Source: three-view drawing plus pictorial views. Frame: mm from the lowest corner of the part. A direction names the side the tool comes from. Give positions to 0.01 mm unless a question says otherwise; leave off trailing zeros. Loops run counter-clockwise (first coordinate to the right, second up) from the corner with the lowest first, then second, coordinate; pieces in that order, holes last.
1. First-contact query: P1, Ø6, axis at x = 48.5, y = 18, coming from the +Z side; P2, Ø1.5, axis at x = 25, y = 12.5, coming from the +Z side; P3, Ø2, axis at x = 42, z = 2, coming from the -Y side; P4, Ø2, axis at x = 16, z = 4.5, coming from the +Y side. Flat tips, straight axial feed; report the tip coordinate or a pass-through.
2. Access query for the marked faces 1, 2, 3 and 4. Directions: +Z, -Z, +X, -X, +Y, -Y. A direction counts if a zero-diameter tool reaches every point of the face in a straight line with its end or side. Return the directions, or none.
3. Section A-A, the plane x = 3.5. Output: boundary loops of the cut face in (y, z), then the cut area to 3 significant figures.
4. Draft query along X for the marked faces 5, 6, 7 and 8. Return one class per face: +X half, -X half, draft (parallel to the pull), parting line (faces both ways), or undercut.
5. Material intervals for line 1 along X through (y, z) = (6.75, 10.25); line 2 along Y through (x, z) = (51.5, 3.5); line 3 along X through (y, z) = (7.5, 5.5), sorted ascending.
6. Section B-B, the plane z = 8.25. Output: boundary loops of the cut face in (x, y).
7. Section D-D, the plane y = 14.75. State how many separate pieces and enclosed holes the cut face has, then the cut area to 3 significant figures.
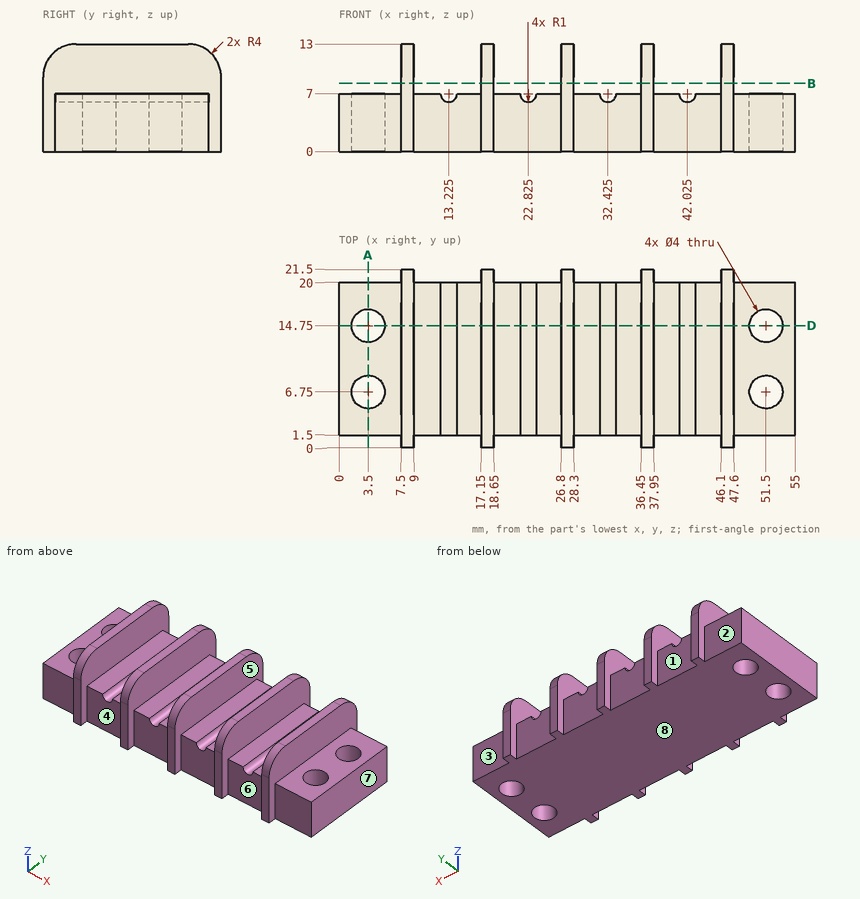
Answers below:
1. P1: stops at z = 13
1. P2: stops at z = 7
1. P3: stops at y = 1.5
1. P4: stops at y = 20
2. face 1: +Z, -Z, +Y
2. face 2: +Z, -Z, -X, +Y
2. face 3: +Z, -Z, +X, +Y
2. face 4: +Z, -Z, -Y
3. outline: (1.5, 0) - (4.75, 0) - (4.75, 7) - (1.5, 7) - close; (8.75, 0) - (12.75, 0) - (12.75, 7) - (8.75, 7) - close; (16.75, 0) - (20, 0) - (20, 7) - (16.75, 7) - close
3. area: 73.5 mm2
4. face 5: undercut
4. face 6: undercut
4. face 7: +X half
4. face 8: draft
5. line 1: x = 7.5 to 9, 17.15 to 18.65, 26.8 to 28.3, 36.45 to 37.95, 46.1 to 47.6
5. line 2: y = 1.5 to 4.75, 8.75 to 12.75, 16.75 to 20
5. line 3: x = 0 to 1.65, 5.35 to 49.65, 53.35 to 55
6. outline: (7.5, 0) - (9, 0) - (9, 21.5) - (7.5, 21.5) - close; (17.15, 0) - (18.65, 0) - (18.65, 21.5) - (17.15, 21.5) - close; (26.8, 0) - (28.3, 0) - (28.3, 21.5) - (26.8, 21.5) - close; (36.45, 0) - (37.95, 0) - (37.95, 21.5) - (36.45, 21.5) - close; (46.1, 0) - (47.6, 0) - (47.6, 21.5) - (46.1, 21.5) - close
7. separate pieces: 3
7. enclosed holes: 0
7. area: 368 mm2
